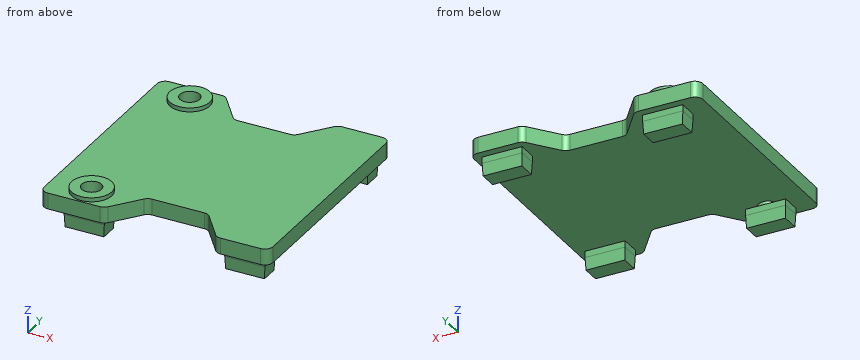
```python
from build123d import *

# Parameters (mm, degrees)
SKETCH1_R                     = 1.575
BOSS_EXTRUDE1_DEPTH           = 2.54
SKETCH2_R                     = 3.175
SKETCH2_R_2                   = 1.575
BOSS_EXTRUDE2_DEPTH           = 0.635
SKETCH3_W                     = 6.35
SKETCH3_H                     = 3
BOSS_EXTRUDE3_DEPTH           = 1
SKETCH4_W                     = 6.35
SKETCH4_H                     = 3
BOSS_EXTRUDE4_DEPTH           = 2
BOSS_EXTRUDE4_DRAFT           = 3
BOSS_EXTRUDE4_PROFILE_2_DEPTH = 2
BOSS_EXTRUDE4_PROFILE_2_DRAFT = 3


with BuildPart() as part:
    # Sketch1 → Boss-Extrude1 (new body)
    with BuildSketch(Plane.XY):
        with BuildLine():
            Line((-184.15, 18.01), (-180.975, 18.01))
            ThreePointArc((-180.975, 18.01), (-180.417860718, 17.88126939), (-179.973667703, 17.521174521))
            Line((-179.973667703, 17.521174521), (-176.593849938, 13.188825479))
            ThreePointArc((-176.593849938, 13.188825479), (-176.149656923, 12.82873061), (-175.592517642, 12.7))
            Line((-175.592517642, 12.7), (-167.307482358, 12.7))
            ThreePointArc((-167.307482358, 12.7), (-166.750343077, 12.82873061), (-166.306150062, 13.188825479))
            Line((-166.306150062, 13.188825479), (-162.926332297, 17.521174521))
            ThreePointArc((-162.926332297, 17.521174521), (-162.482139282, 17.88126939), (-161.925, 18.01))
            Line((-161.925, 18.01), (-155.575, 18.01))
            ThreePointArc((-155.575, 18.01), (-154.676974388, 17.638025612), (-154.305, 16.74))
            Line((-154.305, 16.74), (-154.305, 0))
            Line((-154.305, 0), (-190.5, 0))
            Line((-190.5, 0), (-190.5, 16.74))
            ThreePointArc((-190.5, 16.74), (-190.128025612, 17.638025612), (-189.23, 18.01))
            Line((-189.23, 18.01), (-184.15, 18.01))
        make_face()
        with Locations((-184.15, 14.54645)):
            Circle(SKETCH1_R, mode=Mode.SUBTRACT)
    extrude(amount=BOSS_EXTRUDE1_DEPTH)

    # Sketch2 → Boss-Extrude2 (add)
    with BuildSketch(Plane.XY.offset(2.54)):
        with Locations((-184.15, 14.54645)):
            Circle(SKETCH2_R)
        with Locations((-184.15, 14.54645)):
            Circle(SKETCH2_R_2, mode=Mode.SUBTRACT)
    extrude(amount=BOSS_EXTRUDE2_DEPTH)

    # Sketch3 → Boss-Extrude3 (add)
    with BuildSketch(Plane(origin=(0, 0, 0), x_dir=(-1, 0, 0), z_dir=(0, 0, -1))):
        with Locations((184.15, 15.24)):
            Rectangle(SKETCH3_W, SKETCH3_H)
        with Locations((158.75, 15.24)):
            Rectangle(SKETCH3_W, SKETCH3_H)
    extrude(amount=BOSS_EXTRUDE3_DEPTH)


with BuildPart() as boss_extrude4_tool:
    # Sketch4 → Boss-Extrude4 (with draft: the straight prism first)
    with BuildSketch(Plane(origin=(0, 0, -1), x_dir=(-1, 0, 0), z_dir=(0, 0, -1))):
        with Locations((184.15, 15.24)):
            Rectangle(SKETCH4_W, SKETCH4_H)
    extrude(amount=BOSS_EXTRUDE4_DEPTH)
    # Boss-Extrude4: the draft: its side faces are tilted about the plane it starts from
    boss_extrude4_sides = [boss_extrude4_tool.faces().sort_by_distance(p)[0] for p in [
        (-180.975, 15.24, -2),
        (-184.15, 13.74, -2),
        (-187.325, 15.24, -2),
        (-184.15, 16.74, -2),
    ]]
    draft(boss_extrude4_sides, Plane(origin=(0, 0, -1), x_dir=(-1, 0, 0), z_dir=(0, 0, -1)), BOSS_EXTRUDE4_DRAFT)


with BuildPart() as part_1:
    add(part.part)

    # Boss-Extrude4: add boss_extrude4_tool
    add(boss_extrude4_tool.part)


with BuildPart() as boss_extrude4_profile_2_tool:
    # Sketch4 → Boss-Extrude4 profile 2 (with draft: the straight prism first)
    with BuildSketch(Plane(origin=(0, 0, -1), x_dir=(-1, 0, 0), z_dir=(0, 0, -1))):
        with Locations((158.75, 15.24)):
            Rectangle(SKETCH4_W, SKETCH4_H)
    extrude(amount=BOSS_EXTRUDE4_PROFILE_2_DEPTH)
    # Boss-Extrude4 profile 2: the draft: its side faces are tilted about the plane it starts from
    boss_extrude4_profile_2_sides = [boss_extrude4_profile_2_tool.faces().sort_by_distance(p)[0] for p in [
        (-155.575, 15.24, -2),
        (-158.75, 13.74, -2),
        (-161.925, 15.24, -2),
        (-158.75, 16.74, -2),
    ]]
    draft(boss_extrude4_profile_2_sides, Plane(origin=(0, 0, -1), x_dir=(-1, 0, 0), z_dir=(0, 0, -1)), BOSS_EXTRUDE4_PROFILE_2_DRAFT)


with BuildPart() as part_2:
    add(part_1.part)

    # Boss-Extrude4 profile 2: add boss_extrude4_profile_2_tool
    add(boss_extrude4_profile_2_tool.part)

    # Mirror1: part across plane


with BuildPart() as part_3:
    add(part_2.part)
    add(part_2.part.mirror(Plane.ZX))


solid = part_3.part
```
The listing builds one solid part. Answer for the finished solid, in the listing's coordinates (mm). Round coordinates to 2 decimals unless told otherwise and drop trailing zeros. Write each loop counter-clockwise with the first axis right and the second up, starting at its lowest first coordinate (ties: lowest second). Pieces come first, ordered by that corner, then holes. Notation, with made-up numbers: (-13, -5) -> (28, -5) arc R15 ccw to (28, 7) -> close; hole circle Ø11 at (25.25, -8). An arc over 180 degrees is marked (long way). Answer as a JSON object with one key per item and string values. Group by question number.
Q1. Section C-C (z = 1) is taken. Write down the section's boundary in (x, y) (3 decimals).
Q2. Section D-D (y = -0.5) is taken. Write down the section's boundary in (x, z) (3 decimals), plus the area to 3 significant figures.
Q3. Section B-B (x = -161) is taken. Write down the section's boundary in (y, z), plus the area to 3 significant figures.
Q4. Section A-A (x = -184.15) is taken. Count the separate pieces of the cut face and the enclosed holes in it, plus the area to 3 significant figures.
Q5. Straight lines are drawn through the part: line 1 along Y through (x, z) = (-184.15, 1.6); line 2 along X through (y, z) = (-15.5, 2.5) (3 decimals); line 3 along X through (y, z) = (16, -0.75) (3 decimals). For each, find the intervals that lie inside material, in ascending order.
Q6. Each of these flat-tipped pins is pushed along its axis until it touches: pin 1 Ø8 at (x, y) = (-170, -13) entering from -Z; pin 2 Ø5 at (x, y) = (-167.5, -9.5) entering from +Z; pin 3 Ø3 at (x, z) = (-171.5, 0.5) entering from +Y. Where does it stop, or does it pass through?
Check values:
{
 "1": {"outline": "(-190.5, -16.74) arc R1.27 ccw to (-189.23, -18.01) -> (-180.975, -18.01) arc R1.27 ccw to (-179.974, -17.521) -> (-176.594, -13.189) arc R1.27 cw to (-175.593, -12.7) -> (-167.307, -12.7) arc R1.27 cw to (-166.306, -13.189) -> (-162.926, -17.521) arc R1.27 ccw to (-161.925, -18.01) -> (-155.575, -18.01) arc R1.27 ccw to (-154.305, -16.74) -> (-154.305, 16.74) arc R1.27 ccw to (-155.575, 18.01) -> (-161.925, 18.01) arc R1.27 ccw to (-162.926, 17.521) -> (-166.306, 13.189) arc R1.27 cw to (-167.307, 12.7) -> (-175.593, 12.7) arc R1.27 cw to (-176.594, 13.189) -> (-179.974, 17.521) arc R1.27 ccw to (-180.975, 18.01) -> (-189.23, 18.01) arc R1.27 ccw to (-190.5, 16.74) -> close; hole circle Ø3.15 at (-184.15, -14.546); hole circle Ø3.15 at (-184.15, 14.546)"},
 "2": {"outline": "(-190.5, 0) -> (-154.305, 0) -> (-154.305, 2.54) -> (-190.5, 2.54) -> close", "area": "91.9 mm^2"},
 "3": {"outline": "(-18.01, 0) -> (-16.74, 0) -> (-16.74, -1) -> (-16.64, -3) -> (-13.84, -3) -> (-13.74, -1) -> (-13.74, 0) -> (13.74, 0) -> (13.74, -1) -> (13.84, -3) -> (16.64, -3) -> (16.74, -1) -> (16.74, 0) -> (18.01, 0) -> (18.01, 2.54) -> (-18.01, 2.54) -> close", "area": "109 mm^2"},
 "4": {"separate pieces": "3", "enclosed holes": "0", "area": "97.1 mm^2"},
 "5": {"line 1": "-18.01 to -16.12, -12.97 to 12.97, 16.12 to 18.01", "line 2": "-190.5 to -185.404, -182.896 to -178.397, -164.503 to -154.305", "line 3": "-187.325 to -180.975, -161.925 to -155.575"},
 "6": {"pin 1": "z = 0", "pin 2": "z = 2.54", "pin 3": "y = 12.7"}
}
